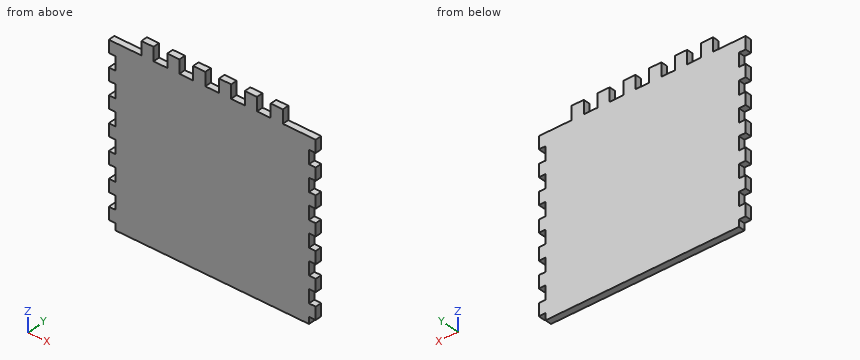
```python
from build123d import *

# Parameters (mm, degrees)
SKETCH1_W           = 101.6
SKETCH1_H           = 107.95
BOSS_EXTRUDE1_DEPTH = 3.175
SKETCH2_W           = 3.302
SKETCH2_H           = 6.604
CUT_EXTRUDE1_DEPTH  = 75.189091179


with BuildPart() as part:
    # Sketch1 → Boss-Extrude1 (new body)
    with BuildSketch(Plane(origin=(0, 0, 0), x_dir=(1, 0, 0), z_dir=(0, 1, 0))):
        Rectangle(SKETCH1_W, SKETCH1_H)
    extrude(amount=BOSS_EXTRUDE1_DEPTH)

    # Sketch2 → Cut-Extrude1 (cut, through all)
    with BuildSketch(Plane.XZ):
        Polygon((-34.798, 31.623), (-47.498, 31.623), (-50.8, 31.623), (-50.8, 38.227), (-50.8, 53.975), (50.8, 53.975), (50.8, 38.227), (50.8, 31.623), (47.498, 31.623), (34.671, 31.623), (34.671, 38.227), (28.702, 38.227), (28.702, 31.623), (21.971, 31.623), (21.971, 38.227), (16.002, 38.227), (16.002, 31.623), (9.271, 31.623), (9.271, 38.227), (3.302, 38.227), (3.302, 31.623), (-3.429, 31.623), (-3.429, 38.227), (-9.398, 38.227), (-9.398, 31.623), (-16.129, 31.623), (-16.129, 38.227), (-22.098, 38.227), (-22.098, 31.623), (-28.829, 31.623), (-28.829, 38.227), (-34.798, 38.227), align=None)
        with Locations((49.149, 22.225)):
            Rectangle(SKETCH2_W, SKETCH2_H)
        with Locations((49.149, 9.525)):
            Rectangle(SKETCH2_W, SKETCH2_H)
        with Locations((49.149, -3.175)):
            Rectangle(SKETCH2_W, SKETCH2_H)
        with Locations((49.149, -15.875)):
            Rectangle(SKETCH2_W, SKETCH2_H)
        with Locations((49.149, -28.575)):
            Rectangle(SKETCH2_W, SKETCH2_H)
        with Locations((49.149, -41.275)):
            Rectangle(SKETCH2_W, SKETCH2_H)
        with Locations((49.149, -53.975)):
            Rectangle(SKETCH2_W, SKETCH2_H)
        with Locations((-49.149, -53.975)):
            Rectangle(SKETCH2_W, SKETCH2_H)
        with Locations((-49.149, -41.275)):
            Rectangle(SKETCH2_W, SKETCH2_H)
        with Locations((-49.149, -28.575)):
            Rectangle(SKETCH2_W, SKETCH2_H)
        with Locations((-49.149, -15.875)):
            Rectangle(SKETCH2_W, SKETCH2_H)
        with Locations((-49.149, -3.175)):
            Rectangle(SKETCH2_W, SKETCH2_H)
        with Locations((-49.149, 9.525)):
            Rectangle(SKETCH2_W, SKETCH2_H)
        with Locations((-49.149, 22.225)):
            Rectangle(SKETCH2_W, SKETCH2_H)
    extrude(amount=-CUT_EXTRUDE1_DEPTH, mode=Mode.SUBTRACT)


solid = part.part
```
Work out the finished part from the listing and answer in its coordinate system (mm). Give positions to 0.01 mm unless a question says otherwise; leave off trailing zeros. Order: outer loops, then holes, each group sorted by start corner. A loop starts at its lowest first (then second) coordinate and runs counter-clockwise, first axis right, second up. Notation, with made-up numbers: (52.5, 38) -> (62.5, 38) arc R17 ccw to (62.5, 45) -> close; hole circle Ø5 at (-4.75, 44.25). An arc over 180 degrees is marked (long way). Answer as CSV lines item,"result". Start each with the question number.
(1) Section A-A, the plane z = -17 is taken. Write down the section's boundary in (x, y) (3 decimals), plus the area to 3 significant figures.
(2) Consider line 1 along Z through (x, y) = (-12.5, 0.4) (3 decimals); line 2 along X through (y, z) = (3, -30.5). Determine where each line is inside the solid, lowest interval first.
(3) Section B-B, the plane x = -25 is taken. Write down the section's boundary in (y, z) (3 decimals), plus the area to 3 significant figures.
(4) Each of these flat-tipped pins is pushed along its axis until it touches: pin 1 Ø1.6 at (y, z) = (2, -4.5) entering from -X; pin 2 Ø1.6 at (x, y) = (50, 1.5) entering from +Z; pin 3 Ø1.6 at (y, z) = (2, 34.5) entering from -X. Where does it stop, or does it pass through?
Entries:
1,outline,"(-47.498, 0) -> (47.498, 0) -> (47.498, 3.175) -> (-47.498, 3.175) -> close"
1,area,"302 mm²"
2,line 1,"-53.975 to 31.623"
2,line 2,"-47.5 to 47.5"
3,outline,"(0, -53.975) -> (3.175, -53.975) -> (3.175, 31.623) -> (0, 31.623) -> close"
3,area,"272 mm²"
4,pin 1,"x = -47.5"
4,pin 2,"z = 31.62"
4,pin 3,"x = -34.8"
